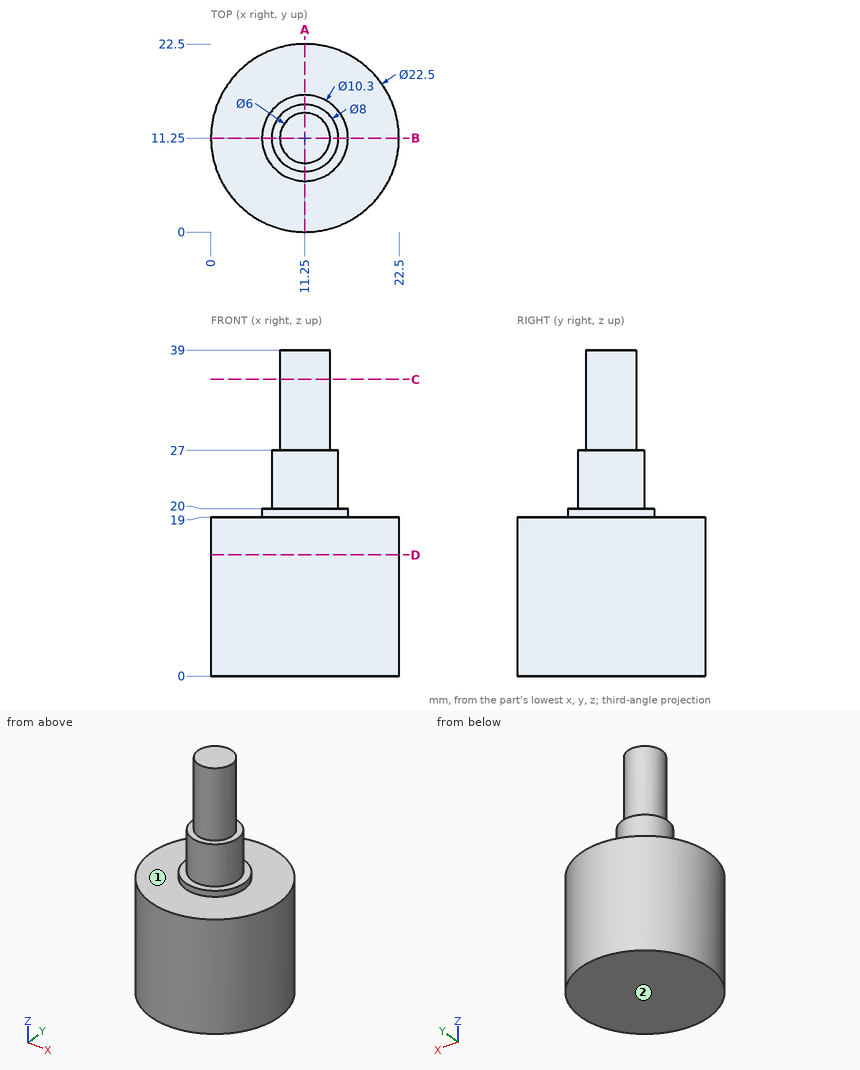
Here's the drawing with two shaded views (mm, measured from the low corner). I have some questions. A direction names the side the tool comes from. Coordinates: 2 decimals unless noted, no trailing zeros. Order: outer loops, then holes, each group sorted by start corner. A loop starts at its lowest first (then second) coordinate and runs counter-clockwise, first axis right, second up.
Q1. Which directions (+Z, -Z, +X, -X, +Y, -Y) give clear straight access to the entire face, cutting with the end or side of a thin tool? Please do the marked faces 1 and 2.
Q2. Please list where these lines run through material, in increasing order: L1, parallel to Y at x = 11.5, z = 28; L2, parallel to Z at x = 18.5, y = 9.25; L3, parallel to Z at x = 12.75, y = 15.
Q3. Suppose I cut it at C-C on z = 35.5. Please give me the cut outline in (x, y).
Q4. Will these pins go through, and if not, where does the flat tip stop? pin 1 (5 mm diameter, centred on x = 19, z = 11.5, fed in from +Y); pin 2 (1 mm diameter, centred on x = 6.5, z = 18, fed in from +Y); pin 3 (4 mm diameter, centred on y = 18.5, z = 20, fed in from -X).
Q5. Suppose I cut it at D-D on z = 14.5. Please give me the cut outline in (x, y), and give its area (3 significant figures).
Q6. Suppose I cut it at A-A on x = 11.25. Please give me the cut outline in (y, z).
Answer:
1. face 1: +Z
1. face 2: -Z, +X, -X, +Y, -Y
2. L1: y = 8.26 to 14.24
2. L2: z = 0 to 19
2. L3: z = 0 to 20
3. outline: circle Ø6 at (11.25, 11.25)
4. pin 1: stops at y = 21.2
4. pin 2: stops at y = 21.67
4. pin 3: stops at x = 1.45
5. outline: circle Ø22.5 at (11.25, 11.25)
5. area: 398 mm2
6. outline: (0, 0) - (22.5, 0) - (22.5, 19) - (16.4, 19) - (16.4, 20) - (15.25, 20) - (15.25, 27) - (14.25, 27) - (14.25, 39) - (8.25, 39) - (8.25, 27) - (7.25, 27) - (7.25, 20) - (6.1, 20) - (6.1, 19) - (0, 19) - close
